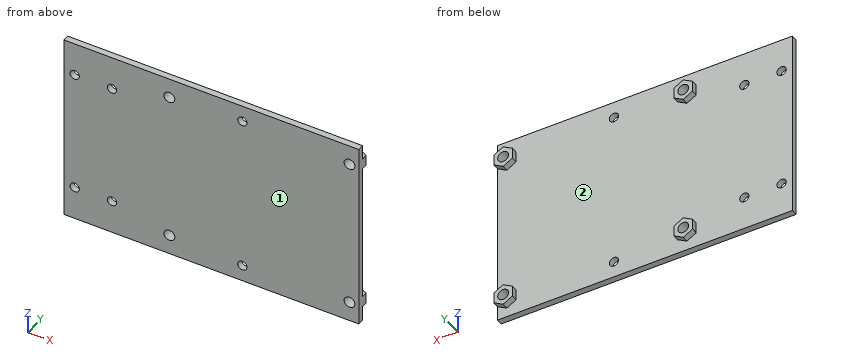
from build123d import *

# Parameters (mm, degrees)
CROQUIS1_W              = 95
CROQUIS1_H              = 62
CROQUIS1_R              = 1.75
CROQUIS1_R_2            = 1.5
SALIENTE_EXTRUIR1_DEPTH = 2
CROQUIS1_4_R            = 1.75
SALIENTE_EXTRUIR2_DEPTH = 4


with BuildPart() as part:
    # Croquis1 → Saliente-Extruir1 (new body)
    with BuildSketch(Plane(origin=(0, 0, 0), x_dir=(1, 0, 0), z_dir=(0, 1, 0))):
        Rectangle(CROQUIS1_W, CROQUIS1_H)
        with Locations(Location((44.5, -24.5, 0), (0, 0, 270))):
            Circle(CROQUIS1_R, mode=Mode.SUBTRACT)
        with Locations(Location((44.5, 24.5, 0), (0, 0, 270))):
            Circle(CROQUIS1_R, mode=Mode.SUBTRACT)
        with Locations(Location((10, 25.63, 0), (0, 0, 270))):
            Circle(CROQUIS1_R_2, mode=Mode.SUBTRACT)
        with Locations(Location((10, -25.63, 0), (0, 0, 270))):
            Circle(CROQUIS1_R_2, mode=Mode.SUBTRACT)
        with Locations(Location((-43.99, 20, 0), (0, 0, 270))):
            Circle(CROQUIS1_R_2, mode=Mode.SUBTRACT)
        with Locations(Location((-31.99, 20, 0), (0, 0, 270))):
            Circle(CROQUIS1_R_2, mode=Mode.SUBTRACT)
        with Locations(Location((-43.99, -20, 0), (0, 0, 270))):
            Circle(CROQUIS1_R_2, mode=Mode.SUBTRACT)
        with Locations(Location((-31.99, -20, 0), (0, 0, 270))):
            Circle(CROQUIS1_R_2, mode=Mode.SUBTRACT)
        with Locations(Location((-13.5, 24.5, 0), (0, 0, 270))):
            Circle(CROQUIS1_R, mode=Mode.SUBTRACT)
        with Locations(Location((-13.5, -24.5, 0), (0, 0, 270))):
            Circle(CROQUIS1_R, mode=Mode.SUBTRACT)
    extrude(amount=SALIENTE_EXTRUIR1_DEPTH)

    # Croquis1_4 → Saliente-Extruir2 (add)
    # profile 1 of 4: a face of its own
    with BuildSketch(Plane(origin=(0, 0, 0), x_dir=(1, 0, 0), z_dir=(0, 1, 0))):
        Polygon((-16.5, 22.767949192), (-13.5, 21.035898385), (-10.5, 22.767949192), (-10.5, 26.232050808), (-13.5, 27.964101615), (-16.5, 26.232050808), align=None)
        with Locations(Location((-13.5, 24.5, 0), (0, 0, 270))):
            Circle(CROQUIS1_4_R, mode=Mode.SUBTRACT)
    # profile 2 of 4: a face of its own
    with BuildSketch(Plane(origin=(0, 0, 0), x_dir=(1, 0, 0), z_dir=(0, 1, 0))):
        Polygon((-16.5, -26.232050808), (-13.5, -27.964101615), (-10.5, -26.232050808), (-10.5, -22.767949192), (-13.5, -21.035898385), (-16.5, -22.767949192), align=None)
        with Locations(Location((-13.5, -24.5, 0), (0, 0, 270))):
            Circle(CROQUIS1_4_R, mode=Mode.SUBTRACT)
    # profile 3 of 4: a face of its own
    with BuildSketch(Plane(origin=(0, 0, 0), x_dir=(1, 0, 0), z_dir=(0, 1, 0))):
        Polygon((44.5, -27.964101615), (47.5, -26.232050808), (47.5, -22.767949192), (44.5, -21.035898385), (41.5, -22.767949192), (41.5, -26.232050808), align=None)
        with Locations(Location((44.5, -24.5, 0), (0, 0, 270))):
            Circle(CROQUIS1_4_R, mode=Mode.SUBTRACT)
    # profile 4 of 4: a face of its own
    with BuildSketch(Plane(origin=(0, 0, 0), x_dir=(1, 0, 0), z_dir=(0, 1, 0))):
        Polygon((47.5, 22.767949192), (47.5, 26.232050808), (44.5, 27.964101615), (41.5, 26.232050808), (41.5, 22.767949192), (44.5, 21.035898385), align=None)
        with Locations(Location((44.5, 24.5, 0), (0, 0, 270))):
            Circle(CROQUIS1_4_R, mode=Mode.SUBTRACT)
    extrude(amount=SALIENTE_EXTRUIR2_DEPTH)


solid = part.part
For this review, take the finished solid that the model builds, in its own axes (mm). Face numbers are marked on the shaded views. A direction names the side the tool comes from. Coordinates: 2 decimals unless noted, no trailing zeros. Loops run counter-clockwise (first coordinate to the right, second up) from the corner with the lowest first, then second, coordinate; pieces in that order, holes last. Notation, with made-up numbers: (37, -38) - (76, -38) arc R18 cw to (76, -3) - close; hole circle Ø5 at (-3.5, 53.25). An arc over 180 degrees is marked (long way). Return JSON: item names as keys, results as strings.
Item 1: For the marked faces 1 and 2, list the 3-axis set-ups (+Z, -Z, +X, -X, +Y, -Y) from which the entire face can be reached by the end or side of a thin tool; tool diameter is ignored.
Determined:
{"face 1": "+Z, -Z, +X, -X, -Y", "face 2": "+Y"}
Item 2: Take a section at A-A (y = 2.9). Give the boundary of the cut face in (x, z).
Determined:
{"outline": "(-16.5, -26.23) - (-13.5, -27.96) - (-10.5, -26.23) - (-10.5, -22.77) - (-13.5, -21.04) - (-16.5, -22.77) - close; (-16.5, 22.77) - (-13.5, 21.04) - (-10.5, 22.77) - (-10.5, 26.23) - (-13.5, 27.96) - (-16.5, 26.23) - close; (41.5, -26.23) - (44.5, -27.96) - (47.5, -26.23) - (47.5, -22.77) - (44.5, -21.04) - (41.5, -22.77) - close; (41.5, 22.77) - (44.5, 21.04) - (47.5, 22.77) - (47.5, 26.23) - (44.5, 27.96) - (41.5, 26.23) - close; hole circle Ø3.5 at (-13.5, -24.5); hole circle Ø3.5 at (-13.5, 24.5); hole circle Ø3.5 at (44.5, -24.5); hole circle Ø3.5 at (44.5, 24.5)"}
Item 3: Take a section at D-D (x = -25). Give the boundary of the cut face in (y, z).
Determined:
{"outline": "(0, -31) - (2, -31) - (2, 31) - (0, 31) - close"}
Item 4: Take a section at B-B (x = -43.99). Give the boundary of the cut face in (y, z).
Determined:
{"outline": "(0, -31) - (2, -31) - (2, -21.5) - (0, -21.5) - close; (0, -18.5) - (2, -18.5) - (2, 18.5) - (0, 18.5) - close; (0, 21.5) - (2, 21.5) - (2, 31) - (0, 31) - close"}
Item 5: For line 1 (X direction, y = 0.6, z = -20); line 2 (X direction, y = 0.4, z = 25.63); line 3 (Y direction, x = 17, z = 22), list the stretches that pass through material, from the lowest coordinate up.
Determined:
{"line 1": "x = -47.5 to -45.49, -42.49 to -33.49, -30.49 to 47.5", "line 2": "x = -47.5 to -14.84, -12.16 to 8.5, 11.5 to 43.16, 45.84 to 47.5", "line 3": "y = 0 to 2"}
Item 6: Insertion check: pin 1 (1 mm diameter, centred on y = 3.5, z = 24, fed in from -X); pin 2 (2.5 mm diameter, centred on x = -43.99, z = 20, fed in from -Y); pin 3 (5 mm diameter, centred on x = 10, z = 25.63, fed in from +Y). Each pin has a flat end and moves straight along its axis. Give the tip position at first contact, or say it passes through.
Determined:
{"pin 1": "stops at x = -16.5", "pin 2": "passes through", "pin 3": "stops at y = 2"}
Item 7: Take a section at C-C (z = -13.5). Give the boundary of the cut face in (x, y), then the cut area to 3 significant figures.
Determined:
{"outline": "(-47.5, 0) - (47.5, 0) - (47.5, 2) - (-47.5, 2) - close", "area": "190 mm2"}
